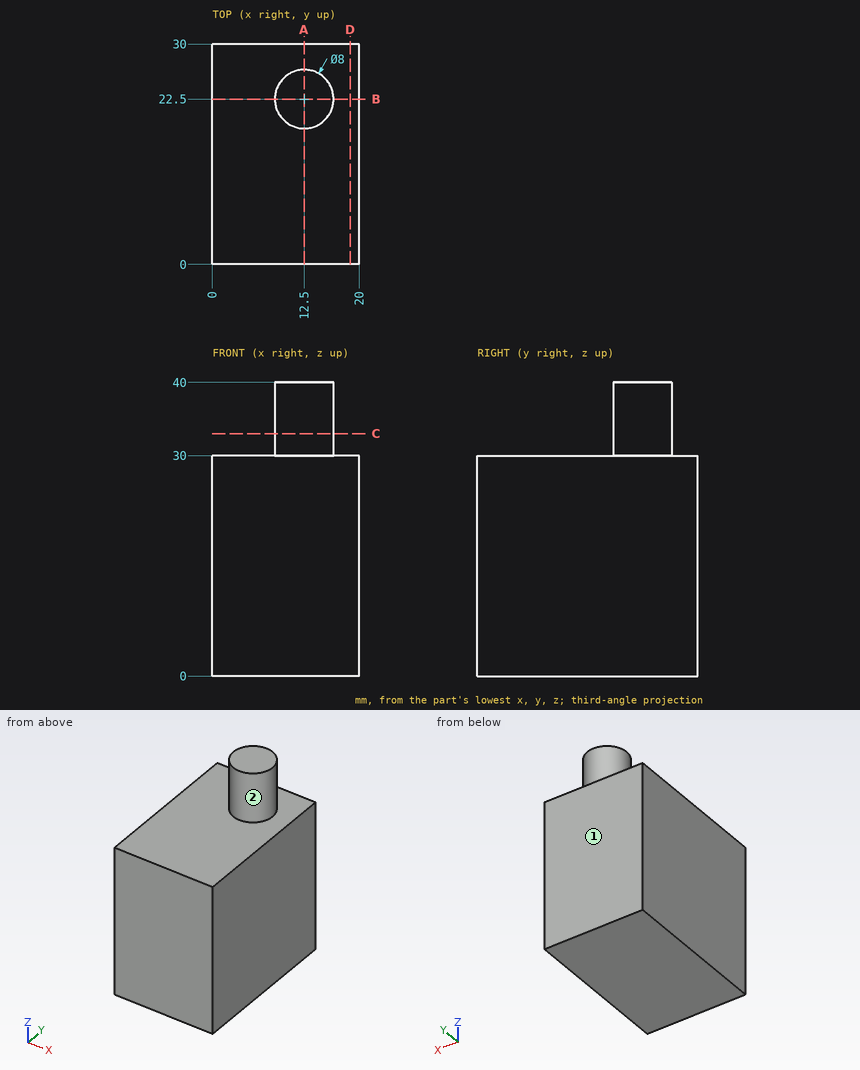
Study the drawing (mm; zero at the part's minimum x, y, z) and answer. A direction names the side the tool comes from. Give positions to 0.01 mm unless a question says otherwise; leave off trailing zeros. Write each loop counter-clockwise with the first axis right and the second up, starting at its lowest first coordinate (ties: lowest second). Pieces come first, ordered by that corner, then holes.
Item 1: Find the intervals of material crossed by line 1 along Z through (x, y) = (19, 6.25); line 2 along Y through (x, z) = (10.5, 37.5); line 3 along X through (y, z) = (22, 38.5), in increasing order.
Item 2: Flat-ended cylindrical pins translate along their axes: P1, Ø1.5, axis at y = 18.5, z = 36, coming from the +X side; P2, Ø1.5, axis at x = 6.5, y = 16, coming from the +Z side. Find the tip coordinate at first contact, or state that the pin passes through.
Item 3: Section C-C, the plane z = 33 is taken. Write down the section's boundary in (x, y).
Item 4: Which of the six approach directions +Z, -Z, +X, -X, +Y, -Y give full straight-line access (tool end or side, diameter ignored) to the marked faces 1 and 2?
Item 5: Section A-A, the plane x = 12.5 is taken. Write down the section's boundary in (y, z), plus the area to 3 significant figures.
Item 6: Section D-D, the plane x = 18.75 is taken. Write down the section's boundary in (y, z), plus the area to 3 significant figures.
Item 7: Section B-B, the plane y = 22.5 is taken. Write down the section's boundary in (x, z), plus the area to 3 significant figures.
Completed:
1. line 1: z = 0 to 30
1. line 2: y = 19.04 to 25.96
1. line 3: x = 8.53 to 16.47
2. P1: stops at x = 14.83
2. P2: stops at z = 30
3. outline: circle Ø8 at (12.5, 22.5)
4. face 1: +Z, -Z, +X, -X, +Y
4. face 2: +Z
5. outline: (0, 0) - (30, 0) - (30, 30) - (26.5, 30) - (26.5, 40) - (18.5, 40) - (18.5, 30) - (0, 30) - close
5. area: 980 mm2
6. outline: (0, 0) - (30, 0) - (30, 30) - (0, 30) - close
6. area: 900 mm2
7. outline: (0, 0) - (20, 0) - (20, 30) - (16.5, 30) - (16.5, 40) - (8.5, 40) - (8.5, 30) - (0, 30) - close
7. area: 680 mm2
